Design review of the part built by this model. Coordinates are the model's own, in mm. Face numbers are marked on the shaded views. Round coordinates to 2 decimals unless told otherwise and drop trailing zeros. Order: outer loops, then holes, each group sorted by start corner. A loop starts at its lowest first (then second) coordinate and runs counter-clockwise, first axis right, second up. Notation, with made-up numbers: M -34.75,-6.75 L -1.75,-6.75 A31 cw -1.75,32.25 Z; hole C 70,-31.5 d11. An arc over 180 degrees is marked long. Use a Markdown table: item, result. Add a question column.
(1) For pin 1 (3 mm diameter, centred on y = 11.5, z = 6, fed in from +X), flat-tipped, find the tip position at first contact; note if it passes through.
(2) Take a section at D-D (x = 22). Write out the cut boundary in (y, z), then the cut area to 3 significant figures.
(3) The part is to be moulded in two halves that separate along Y. For the marked faces 1, 2, 3 and 4, say which applies: released by +Y, released by -Y, zero draft, split by the parting line, or undercut.
(4) To check wall thickness, follow probe 1 along X at (y, z) = (-1.5, 2); probe 2 along X at (y, z) = (7, 6); probe 3 along Y at (x, z) = (0.5, 5.75). State the ranges of each line that lie inside material, in increasing order. Write a range as from..to.
(5) Take a section at C-C (z = 3). Write out the cut boundary in (x, y).
(6) Take a section at A-A (y = 0). Count the separate pieces of the cut face and the enclosed holes in it, then the cut area to 3 significant figures.
```python
from build123d import *

# Parameters (mm, degrees)
F0_R     = 11.2
F1_DEPTH = 9
F2_R     = 3.6213203436
F3_R     = 4.99999


# Not quite as in the source:
# - a fillet or chamfer is up to 0.001 mm smaller than in the source, because OpenCascade refuses the exact size


with BuildPart() as f1:
    # F0 (on Top) → F1 (new body)
    with BuildSketch(Plane.XY):
        with BuildLine():
            Line((28.6, 16.2), (-28.6, 16.2))
            ThreePointArc((-28.6, 16.2), (-39.2066017178, 11.8066017178), (-43.6, 1.2))
            Line((-43.6, 1.2), (-43.6, -1.2))
            ThreePointArc((-43.6, -1.2), (-39.2066017178, -11.8066017178), (-28.6, -16.2))
            Line((-28.6, -16.2), (28.6, -16.2))
            ThreePointArc((28.6, -16.2), (39.2066017178, -11.8066017178), (43.6, -1.2))
            Line((43.6, -1.2), (43.6, 1.2))
            ThreePointArc((43.6, 1.2), (39.2066017178, 11.8066017178), (28.6, 16.2))
        make_face()
        with Locations((-27.4, 0)):
            Circle(F0_R, mode=Mode.SUBTRACT)
        Circle(F0_R, mode=Mode.SUBTRACT)
        with Locations((27.4, 0)):
            Circle(F0_R, mode=Mode.SUBTRACT)
    extrude(amount=F1_DEPTH)

    # F2
    f2_edges = [f1.edges().sort_by_distance(p)[0] for p in [
        (39.206602, 11.806602, 9),
    ]]
    fillet(f2_edges, radius=F2_R)

    # F3 (radius 5 in the source; OpenCascade refuses exactly that, so slightly less here)
    f3_edges = [f1.edges().sort_by_distance(p)[0] for p in [
        (0, 16.2, 0),
        (39.206602, 11.806602, 0),
    ]]
    fillet(f3_edges, radius=F3_R)


solid = f1.part
```
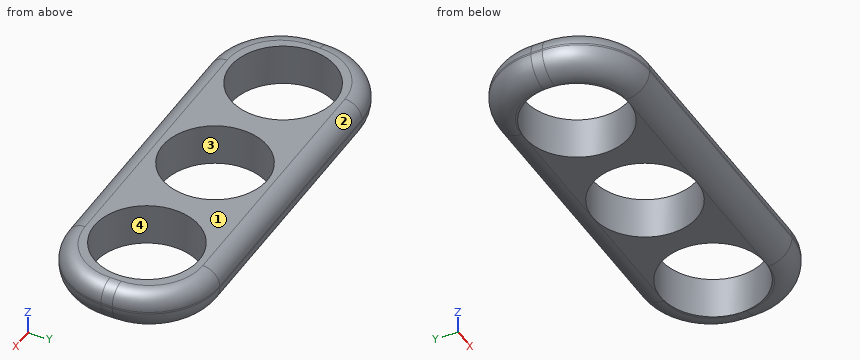
Verdict:
| question | item | result |
|---|---|---|
| 1 | pin 1 | stops at x = 40.71 |
| 2 | outline | M -16.2,5 A5 ccw -11.2,0 L -9.81,0 L -9.81,9 L -12.58,9 A3.62 ccw -16.2,5.38 Z; M 9.81,0 L 11.2,0 A5 ccw 16.2,5 L 16.2,5.38 A3.62 ccw 12.58,9 L 9.81,9 Z |
| 2 | area | 98.6 mm^2 |
| 3 | face 1 | zero draft |
| 3 | face 2 | released by +Y |
| 3 | face 3 | undercut |
| 3 | face 4 | undercut |
| 4 | probe 1 | x = -42.6..-38.5, -16.3..-11.1, 11.1..16.3, 38.5..42.6 |
| 4 | probe 2 | x = -42.38..-36.14, -18.66..-8.74, 8.74..18.66, 36.14..42.38 |
| 4 | probe 3 | y = -16.18..-11.19, 11.19..16.18 |
| 5 | outline | M -43.18,-1.2 A14.58 ccw -28.6,-15.78 L 28.6,-15.78 A14.58 ccw 43.18,-1.2 L 43.18,1.2 A14.58 ccw 28.6,15.78 L -28.6,15.78 A14.58 ccw -43.18,1.2 Z; hole C -27.4,0 d22.4; hole C 0,0 d22.4; hole C 27.4,0 d22.4 |
| 6 | separate pieces | 4 |
| 6 | enclosed holes | 0 |
| 6 | area | 164 mm^2 |
